from build123d import *

# Parameters (mm, degrees)
SKETCH1_R             = 8
SKETCH1_R_2           = 3.75
BOSS_EXTRUDE1_DEPTH   = 20
BOSS_EXTRUDE1_2_DEPTH = 20
BOSS_EXTRUDE2_DEPTH   = 8
SKETCH1_4_R           = 8
SKETCH1_4_R_2         = 3.75
BOSS_EXTRUDE3_DEPTH   = 16
SKETCH3_R             = 3.75
CUT_EXTRUDE2_DEPTH    = 16
SKETCH4_R             = 3.75
CUT_EXTRUDE3_DEPTH    = 16


with BuildPart() as part:
    # Sketch1 → Boss-Extrude1 (new body)
    with BuildSketch(Plane(origin=(0, 0, 0), x_dir=(1, 0, 0), z_dir=(0, 1, 0))):
        with Locations(Location((0, 0, 0), (0, 0, 270))):
            Circle(SKETCH1_R)
        with Locations(Location((0, 0, 0), (0, 0, 270))):
            Circle(SKETCH1_R_2, mode=Mode.SUBTRACT)
    extrude(amount=BOSS_EXTRUDE1_DEPTH)



with BuildPart() as body_2:
    # Sketch1 → Boss-Extrude1 2 (new body)
    with BuildSketch(Plane(origin=(0, 0, 0), x_dir=(1, 0, 0), z_dir=(0, 1, 0))):
        with Locations(Location((-165, 0, 0), (0, 0, 90))):
            Circle(SKETCH1_R)
        with Locations(Location((-165, 0, 0), (0, 0, 90))):
            Circle(SKETCH1_R_2, mode=Mode.SUBTRACT)
    extrude(amount=BOSS_EXTRUDE1_2_DEPTH)


with BuildPart() as part_1:
    add(part.part)

    add(body_2.part)  # Boss-Extrude2 merges body 2
    # Sketch2 → Boss-Extrude2 (add, symmetric)
    with BuildSketch(Plane.XY):
        Polygon((0, 4), (-165, 4), (-165, 11.640611033), (-165, 16), (-157, 16), (-153.819851171, 16), (-152.909925586, 18.5), (-151.909925586, 18.5), (-150.909925586, 18.5), (-150, 16), (-147.819851171, 16), (-146.909925586, 18.5), (-145.909925586, 18.5), (-144.909925586, 18.5), (-144, 16), (-141.819851171, 16), (-140.909925586, 18.5), (-139.909925586, 18.5), (-138.909925586, 18.5), (-138, 16), (-135.819851171, 16), (-134.909925586, 18.5), (-133.909925586, 18.5), (-132.909925586, 18.5), (-132, 16), (-129.819851171, 16), (-128.909925586, 18.5), (-127.909925586, 18.5), (-126.909925586, 18.5), (-126, 16), (-123.819851171, 16), (-122.909925586, 18.5), (-121.909925586, 18.5), (-120.909925586, 18.5), (-120, 16), (-117.819851171, 16), (-116.909925586, 18.5), (-115.909925586, 18.5), (-114.909925586, 18.5), (-114, 16), (-111.819851171, 16), (-110.909925586, 18.5), (-109.909925586, 18.5), (-108.909925586, 18.5), (-108, 16), (-105.819851171, 16), (-104.909925586, 18.5), (-103.909925586, 18.5), (-102.909925586, 18.5), (-102, 16), (-99.819851171, 16), (-98.909925586, 18.5), (-97.909925586, 18.5), (-96.909925586, 18.5), (-96, 16), (-93.819851171, 16), (-92.909925586, 18.5), (-91.909925586, 18.5), (-90.909925586, 18.5), (-90, 16), (-87.819851171, 16), (-86.909925586, 18.5), (-85.909925586, 18.5), (-84.909925586, 18.5), (-84, 16), (-81.819851171, 16), (-80.909925586, 18.5), (-79.909925586, 18.5), (-78.909925586, 18.5), (-78, 16), (-75.819851171, 16), (-74.909925586, 18.5), (-73.909925586, 18.5), (-72.909925586, 18.5), (-72, 16), (-69.819851171, 16), (-68.909925586, 18.5), (-67.909925586, 18.5), (-66.909925586, 18.5), (-66, 16), (-63.819851171, 16), (-62.909925586, 18.5), (-61.909925586, 18.5), (-60.909925586, 18.5), (-60, 16), (-57.819851171, 16), (-56.909925586, 18.5), (-55.909925586, 18.5), (-54.909925586, 18.5), (-54, 16), (-51.819851171, 16), (-50.909925586, 18.5), (-49.909925586, 18.5), (-48.909925586, 18.5), (-48, 16), (-45.819851171, 16), (-44.909925586, 18.5), (-43.909925586, 18.5), (-42.909925586, 18.5), (-42, 16), (-39.819851171, 16), (-38.909925586, 18.5), (-37.909925586, 18.5), (-36.909925586, 18.5), (-36, 16), (-33.819851171, 16), (-32.909925586, 18.5), (-31.909925586, 18.5), (-30.909925586, 18.5), (-30, 16), (-27.819851171, 16), (-26.909925586, 18.5), (-25.909925586, 18.5), (-24.909925586, 18.5), (-24, 16), (-21.819851171, 16), (-20.909925586, 18.5), (-19.909925586, 18.5), (-18.909925586, 18.5), (-18, 16), (-15.819851171, 16), (-14.909925586, 18.5), (-13.909925586, 18.5), (-12.909925586, 18.5), (-12, 16), (0, 16), align=None)
    extrude(amount=BOSS_EXTRUDE2_DEPTH, both=True)

    # Sketch1_4 → Boss-Extrude3 (add)
    # profile 1 of 2: a face of its own
    with BuildSketch(Plane(origin=(0, 0, 0), x_dir=(1, 0, 0), z_dir=(0, 1, 0))):
        with Locations(Location((0, 0, 0), (0, 0, 270))):
            Circle(SKETCH1_4_R)
        with Locations(Location((0, 0, 0), (0, 0, 270))):
            Circle(SKETCH1_4_R_2, mode=Mode.SUBTRACT)
    # profile 2 of 2: a face of its own
    with BuildSketch(Plane(origin=(0, 0, 0), x_dir=(1, 0, 0), z_dir=(0, 1, 0))):
        with Locations(Location((-165, 0, 0), (0, 0, 90))):
            Circle(SKETCH1_4_R)
        with Locations(Location((-165, 0, 0), (0, 0, 90))):
            Circle(SKETCH1_4_R_2, mode=Mode.SUBTRACT)
    extrude(amount=BOSS_EXTRUDE3_DEPTH)

    # Sketch3 → Cut-Extrude2 (cut)
    with BuildSketch(Plane(origin=(0, 0, 0), x_dir=(-1, 0, 0), z_dir=(0, -1, 0))):
        with Locations(Location((165, 0, 0), (0, 0, 90))):
            Circle(SKETCH3_R)
    extrude(amount=-CUT_EXTRUDE2_DEPTH, mode=Mode.SUBTRACT)

    # Sketch4 → Cut-Extrude3 (cut)
    with BuildSketch(Plane(origin=(0, 0, 0), x_dir=(-1, 0, 0), z_dir=(0, -1, 0))):
        with Locations(Location((0, 0, 0), (0, 0, 270))):
            Circle(SKETCH4_R)
    extrude(amount=-CUT_EXTRUDE3_DEPTH, mode=Mode.SUBTRACT)


solid = part_1.part
Geometry check sheet. Reference: the model listing, model coordinates, mm. A direction names the side the tool comes from. Coordinates: 2 decimals unless noted, no trailing zeros. Order: outer loops, then holes, each group sorted by start corner. A loop starts at its lowest first (then second) coordinate and runs counter-clockwise, first axis right, second up. Notation, with made-up numbers: (26.5, -12.75) -> (37.5, -12.75) arc R12 cw to (37.5, -1.75) -> close; hole circle Ø5 at (18.25, -31.75). An arc over 180 degrees is marked (long way). Use a Markdown table: item, result. Add a question column.
1. Set-up check for faces 3 (the face through (-9, 16, 0)), 4 (the face through (0.165, 9.86, -3.746)), 5 (the face through (-172.932, 9.86, 1.041)): record each of +Z, -Z, +X, -X, +Y, -Y from which the full face is reachable in a straight line by a thin tool's end or side.
2. Go/stop test with flat-tipped pins: pin 1 Ø2 at (y, z) = (2.5, -1.5) entering from +X; pin 2 Ø1.5 at (x, z) = (-116.5, -6.5) entering from +Y; pin 3 Ø1 at (x, z) = (-121.5, -0.5) entering from -Y. Record where each tip stops, or that it passes through.
3. Cross-section at A-A (y = 11). Enter the section's corners in (x, z).
4. Material ranges on L1, parallel to X at y = 7.75, z = 0; L2, parallel to X at y = 12.5, z = 2.5; L3, parallel to Z at x = -165, y = 8.25, recorded low to high.
5. Mould release check, pull along X, two halves, no side actions. Record for faces 1 (the face through (1.89, 20, 3.44)), 2 (the face through (7.932, 9.86, -1.041)): pulls with the +X half, pulls with the -X half, needs draft (parallel to the pull), parting line crosses it, or undercut.
6. Cross-section at B-B (z = 0). Give the number of separate pieces and of enclosed holes in the cut face, and give its area (3 significant figures).
Filled sheet:
| question | item | result |
|---|---|---|
| 1 | face 3 | +Y |
| 1 | face 4 | +Y, -Y |
| 1 | face 5 | none |
| 2 | pin 1 | x = 7.98 |
| 2 | pin 2 | y = 18.5 |
| 2 | pin 3 | y = 4 |
| 3 | outline | (-165, -8) -> (0, -8) arc R8 ccw to (0, 8) -> (-165, 8) arc R8 ccw to start; hole circle Ø7.5 at (-165, 0); hole circle Ø7.5 at (0, 0) |
| 4 | L1 | -173 to -168.75, -161.25 to -3.75, 3.75 to 8 |
| 4 | L2 | -172.6 to -167.8, -162.2 to -2.8, 2.8 to 7.6 |
| 4 | L3 | -8 to -3.75, 3.75 to 8 |
| 5 | face 1 | needs draft |
| 5 | face 2 | undercut |
| 6 | separate pieces | 3 |
| 6 | enclosed holes | 0 |
| 6 | area | 2,300 mm2 |
